Could you check a few things on this drawing? It's one solid part, dimensions in mm from its lowest x, y, z. A direction names the side the tool comes from. Coordinates: 2 decimals unless noted, no trailing zeros. Write each loop counter-clockwise with the first axis right and the second up, starting at its lowest first coordinate (ties: lowest second). Pieces come first, ordered by that corner, then holes. Notation, with made-up numbers: M 46,87.5 L 62,87.5 A6 cw 62,92.5 Z; hole C 35,-17 d1. An arc over 180 degrees is marked long. Use a Markdown table: item, result.
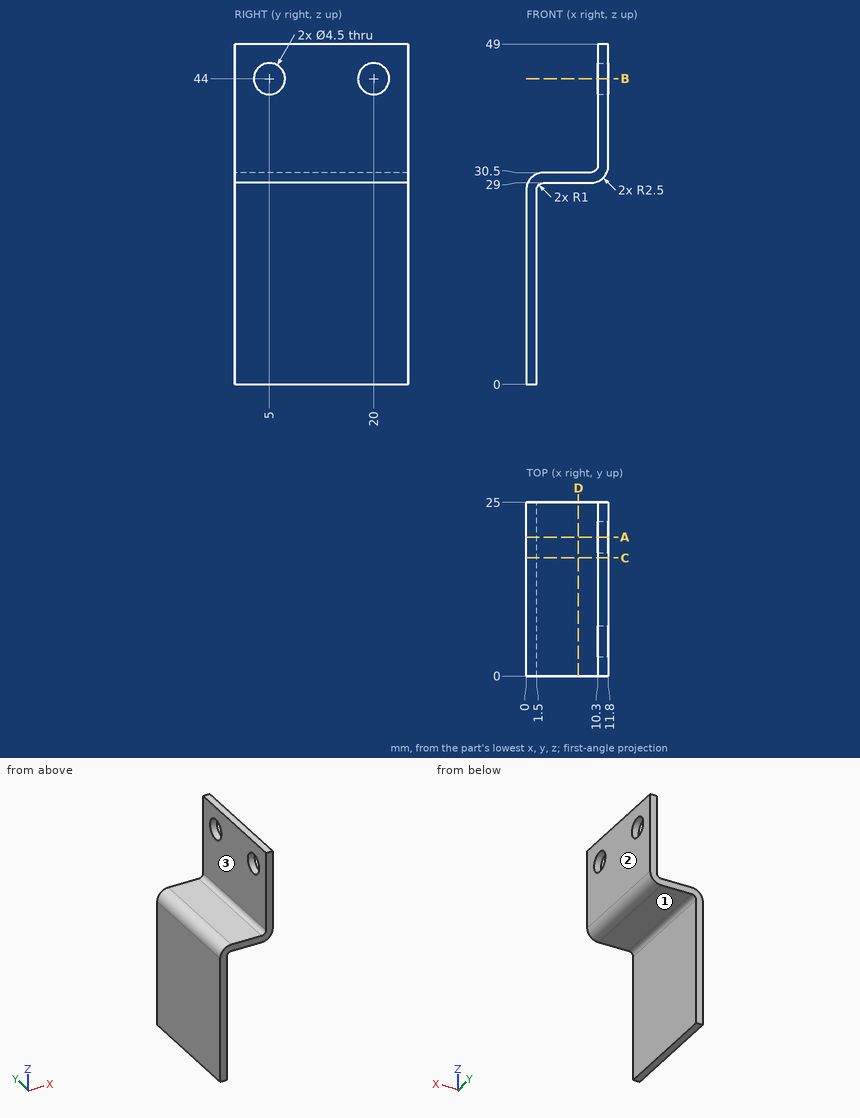
1. Suppose I cut it at A-A on y = 20. Write out the boundary of the cut face in (x, z), and give its area (3 significant figures).
Answers follow:
| item | result |
|---|---|
| outline | M 0,0 L 1.5,0 L 1.5,28 A1 cw 2.5,29 L 9.3,29 A2.5 ccw 11.8,31.5 L 11.8,41.75 L 10.3,41.75 L 10.3,31.5 A1 cw 9.3,30.5 L 2.5,30.5 A2.5 ccw 0,28 Z; M 10.3,46.25 L 11.8,46.25 L 11.8,49 L 10.3,49 Z |
| area | 79.9 mm2 |
2. Suppose I cut it at C-C on y = 17. Write out the boundary of the cut face in (x, z).
Answers follow:
| item | result |
|---|---|
| outline | M 0,0 L 1.5,0 L 1.5,28 A1 cw 2.5,29 L 9.3,29 A2.5 ccw 11.8,31.5 L 11.8,49 L 10.3,49 L 10.3,31.5 A1 cw 9.3,30.5 L 2.5,30.5 A2.5 ccw 0,28 Z |
3. Suppose I cut it at B-B on z = 44. Write out the boundary of the cut face in (x, y), and give its area (3 significant figures).
Answers follow:
| item | result |
|---|---|
| outline | M 10.3,0 L 11.8,0 L 11.8,2.75 L 10.3,2.75 Z; M 10.3,7.25 L 11.8,7.25 L 11.8,17.75 L 10.3,17.75 Z; M 10.3,22.25 L 11.8,22.25 L 11.8,25 L 10.3,25 Z |
| area | 24.0 mm2 |
4. I need wall thicknesses on probe 1 along Y at (x, z) = (10.7, 44); probe 2 along X at (y, z) = (5.5, 4); probe 3 along X at (y, z) = (3.5, 37). Which ranges of each line are inside material? Lowest first, please.
Answers follow:
| item | result |
|---|---|
| probe 1 | y = 0 to 2.75, 7.25 to 17.75, 22.25 to 25 |
| probe 2 | x = 0 to 1.5 |
| probe 3 | x = 10.3 to 11.8 |
5. Will these pins go through, and if not, where does the flat tip stop? pin 1 Ø7 at (y, z) = (20, 44) entering from -X; pin 2 Ø5 at (x, z) = (6.5, 31.5) entering from +Y; pin 3 Ø1.5 at (y, z) = (13.5, 18) entering from +X; pin 4 Ø2 at (x, y) = (6, 15.5) entering from +Z.
Answers follow:
| item | result |
|---|---|
| pin 1 | stops at x = 10.3 |
| pin 2 | stops at y = 25 |
| pin 3 | stops at x = 1.5 |
| pin 4 | stops at z = 30.5 |
6. Suppose I cut it at D-D on x = 7.5. Write out the boundary of the cut face in (y, z), and give its area (3 significant figures).
Answers follow:
| item | result |
|---|---|
| outline | M 0,29 L 25,29 L 25,30.5 L 0,30.5 Z |
| area | 37.5 mm2 |
7. Which directions (+Z, -Z, +X, -X, +Y, -Y) give clear straight access to the entire face, cutting with the end or side of a thin tool? Please do the marked faces 1, 2 and 3.
Answers follow:
| item | result |
|---|---|
| face 1 | -Z, +X, +Y, -Y |
| face 2 | +Z, -Z, +X, +Y, -Y |
| face 3 | +Z, -X, +Y, -Y |
